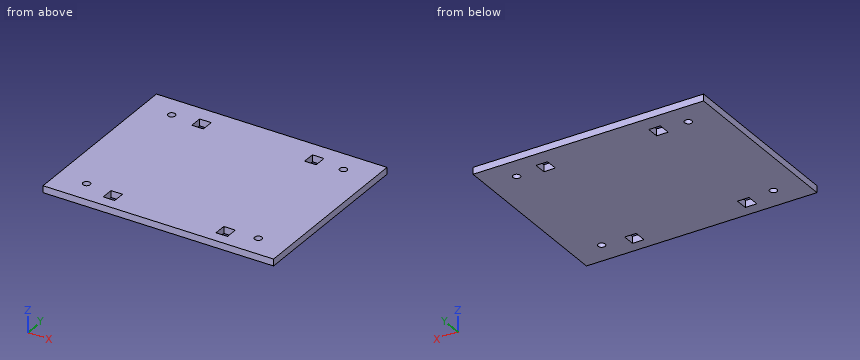
```python
from build123d import *

# Parameters (mm, degrees)
SKETCH_1_W                       = 102
SKETCH_1_H                       = 80
SKETCH_1_R                       = 1.6
EXTRUDE_1_DEPTH                  = 3
SKETCH_4_W                       = 5.1
SKETCH_4_H                       = 5.5
CUT_EXTRUDE_2_DEPTH              = 5
PATTERN_LINEAR_1_COUNT           = 2
PATTERN_LINEAR_1_PITCH           = 62.5
PATTERN_LINEAR_1_COPY_1_SKETCH_W = 5.1
PATTERN_LINEAR_1_COPY_1_SKETCH_H = 5.5
PATTERN_LINEAR_1_COPY_1_DEPTH    = 5


with BuildPart() as part:
    # 草图1 → 凸台-拉伸1 (new body)
    with BuildSketch(Plane.XY):
        with Locations((0, -65.25)):
            Rectangle(SKETCH_1_W, SKETCH_1_H)
        with Locations((-38, -35.25)):
            Circle(SKETCH_1_R, mode=Mode.SUBTRACT)
        with Locations((-38, -95.25)):
            Circle(SKETCH_1_R, mode=Mode.SUBTRACT)
        with Locations((38, -95.25)):
            Circle(SKETCH_1_R, mode=Mode.SUBTRACT)
        with Locations((38, -35.25)):
            Circle(SKETCH_1_R, mode=Mode.SUBTRACT)
    extrude(amount=EXTRUDE_1_DEPTH)

    # 草图4 → 切除-拉伸2 (cut)
    with BuildSketch(Plane.XY.offset(3)):
        with Locations((-24.949999999, -97.5)):
            Rectangle(SKETCH_4_W, SKETCH_4_H)
    cut_extrude_2 = extrude(amount=-CUT_EXTRUDE_2_DEPTH, mode=Mode.SUBTRACT)

    # 镜向1: 切除-拉伸2 across plane
    add(cut_extrude_2.mirror(Plane.ZY), mode=Mode.SUBTRACT)

    # 阵列(线性)1: 切除-拉伸2 ×2
    with Locations(*[(0, i * PATTERN_LINEAR_1_PITCH, 0) for i in range(1, PATTERN_LINEAR_1_COUNT)]):
        add(cut_extrude_2, mode=Mode.SUBTRACT)

    # 阵列(线性)1 copy 1 sketch → 阵列(线性)1 copy 1 (cut)
    with BuildSketch(Plane(origin=(0, 62.5, 3), x_dir=(-1, 0, 0), z_dir=(0, 0, 1))):
        with Locations((-24.949999999, 97.5)):
            Rectangle(PATTERN_LINEAR_1_COPY_1_SKETCH_W, PATTERN_LINEAR_1_COPY_1_SKETCH_H)
    extrude(amount=-PATTERN_LINEAR_1_COPY_1_DEPTH, mode=Mode.SUBTRACT)


solid = part.part
```
Design review of the part built by this model. Coordinates are the model's own, in mm. Give positions to 0.01 mm unless a question says otherwise; leave off trailing zeros. Loops run counter-clockwise (first coordinate to the right, second up) from the corner with the lowest first, then second, coordinate; pieces in that order, holes last. Notation, with made-up numbers: (23.5, 75) -> (32.5, 75) arc R22 ccw to (32.5, 92) -> close; hole circle Ø10 at (26.5, -25). An arc over 180 degrees is marked (long way). One line per item, written item: value.
Q1. We need section B-B on z = 1.6. Give the number of separate pieces and of enclosed holes in the cut face, and give its area (3 significant figures).
Numbers:
separate pieces: 1
enclosed holes: 8
area: 8,020 mm^2
Q2. For L1, parallel to X at y = -95, z = 1.5; L2, parallel to Y at x = -26, z = 2.1; L3, parallel to Y at x = 38, z = 1.75, list the stretches that pass through material, from the lowest coordinate up.
Numbers:
L1: x = -51 to -39.58, -36.42 to -27.5, -22.4 to 22.4, 27.5 to 36.42, 39.58 to 51
L2: y = -105.25 to -100.25, -94.75 to -37.75, -32.25 to -25.25
L3: y = -105.25 to -96.85, -93.65 to -36.85, -33.65 to -25.25
Q3. We need section A-A on x = 38. Give the boundary of the cut face in (y, z), and give its area (3 significant figures).
Numbers:
outline: (-105.25, 0) -> (-96.85, 0) -> (-96.85, 3) -> (-105.25, 3) -> close; (-93.65, 0) -> (-36.85, 0) -> (-36.85, 3) -> (-93.65, 3) -> close; (-33.65, 0) -> (-25.25, 0) -> (-25.25, 3) -> (-33.65, 3) -> close
area: 221 mm^2
